```python
from build123d import *

# Parameters (mm, degrees)
BOSS_EXTRUDE1_DEPTH                             = 182.5
CUT_EXTRUDE1_DEPTH                              = 251
CUT_EXTRUDE2_DEPTH                              = 10
SKETCH4_W                                       = 2
SKETCH4_H                                       = 246
BOSS_EXTRUDE2_DEPTH                             = 43
SKETCH5_W                                       = 3
SKETCH5_H                                       = 3
CUT_EXTRUDE3_DEPTH                              = 46
FILLET1_R                                       = 0.5
FILLET2_R                                       = 2.5
CUT_EXTRUDE6_DEPTH                              = 366
SKETCH9_R                                       = 2.25
CUT_EXTRUDE7_DEPTH                              = 366
SKETCH10_R                                      = 2.25
CUT_EXTRUDE8_DEPTH                              = 10
SKETCH11_R                                      = 2.25
CUT_EXTRUDE9_DEPTH                              = 10
SKETCH12_R                                      = 1.5
CUT_EXTRUDE10_DEPTH                             = 10
CSK_FOR_M3_FLAT_HEAD_MACHINE_SCREW1_D           = 3.4
CSK_FOR_M3_FLAT_HEAD_MACHINE_SCREW1_CSINK_D     = 6.3
CSK_FOR_M3_FLAT_HEAD_MACHINE_SCREW1_CSINK_ANGLE = 90


with BuildPart() as part:
    # Sketch1 → Boss-Extrude1 (new body, symmetric)
    with BuildSketch(Plane(origin=(0, 0, 0), x_dir=(0, 0, -1), z_dir=(1, 0, 0))):
        with BuildLine():
            Line((123, -45), (125, -45))
            Line((125, -45), (125, -2.5))
            ThreePointArc((125, -2.5), (124.267766953, -0.732233047), (122.5, 0))
            Line((122.5, 0), (-122.5, 0))
            ThreePointArc((-122.5, 0), (-124.267766953, -0.732233047), (-125, -2.5))
            Line((-125, -2.5), (-125, -45))
            Line((-125, -45), (-123, -45))
            Line((-123, -45), (-123, -2.5))
            ThreePointArc((-123, -2.5), (-122.853553391, -2.146446609), (-122.5, -2))
            Line((-122.5, -2), (122.5, -2))
            ThreePointArc((122.5, -2), (122.853553391, -2.146446609), (123, -2.5))
            Line((123, -2.5), (123, -45))
        make_face()
    extrude(amount=BOSS_EXTRUDE1_DEPTH, both=True)

    # Sketch2 → Cut-Extrude1 (cut, through all)
    with BuildSketch(Plane.XY.offset(125)):
        with BuildLine():
            Line((-164.5, -45), (164.5, -45))
            Line((164.5, -45), (164.5, -28))
            ThreePointArc((164.5, -28), (161.571067812, -20.928932188), (154.5, -18))
            Line((154.5, -18), (-154.5, -18))
            ThreePointArc((-154.5, -18), (-161.571067812, -20.928932188), (-164.5, -28))
            Line((-164.5, -28), (-164.5, -45))
        make_face()
    extrude(amount=-CUT_EXTRUDE1_DEPTH, mode=Mode.SUBTRACT)

    # Sketch3 → Cut-Extrude2 (cut)
    with BuildSketch(Plane(origin=(0, 0, 0), x_dir=(1, 0, 0), z_dir=(0, 1, 0))):
        with BuildLine():
            Line((-117.5, 105), (117.5, 105))
            ThreePointArc((117.5, 105), (131.642135624, 99.142135624), (137.5, 85))
            Line((137.5, 85), (137.5, -45))
            ThreePointArc((137.5, -45), (131.642135624, -59.142135624), (117.5, -65))
            Line((117.5, -65), (-117.5, -65))
            ThreePointArc((-117.5, -65), (-131.642135624, -59.142135624), (-137.5, -45))
            Line((-137.5, -45), (-137.5, 85))
            ThreePointArc((-137.5, 85), (-131.642135624, 99.142135624), (-117.5, 105))
        make_face()
    extrude(amount=-CUT_EXTRUDE2_DEPTH, mode=Mode.SUBTRACT)

    # Sketch4 → Boss-Extrude2 (add)
    with BuildSketch(Plane.XZ.offset(2)):
        with Locations((-181.5, 0)):
            Rectangle(SKETCH4_W, SKETCH4_H)
        with Locations((181.5, 0)):
            Rectangle(SKETCH4_W, SKETCH4_H)
    extrude(amount=BOSS_EXTRUDE2_DEPTH)

    # Sketch5 → Cut-Extrude3 (cut, through all)
    with BuildSketch(Plane.XZ.offset(45)):
        with Locations((-181, 123.5)):
            Rectangle(SKETCH5_W, SKETCH5_H)
        with Locations((-181, -123.5)):
            Rectangle(SKETCH5_W, SKETCH5_H)
        with Locations((181, -123.5)):
            Rectangle(SKETCH5_W, SKETCH5_H)
        with Locations((181, 123.5)):
            Rectangle(SKETCH5_W, SKETCH5_H)
    extrude(amount=-CUT_EXTRUDE3_DEPTH, mode=Mode.SUBTRACT)

    # Fillet1
    fillet1_edges = [part.edges().sort_by_distance(p)[0] for p in [
        (-180.5, -2, 0),
        (180.5, -2, 0),
    ]]
    fillet(fillet1_edges, radius=FILLET1_R)

    # Fillet2
    fillet2_edges = [part.edges().sort_by_distance(p)[0] for p in [
        (-182.5, 0, 0),
        (182.5, 0, 0),
    ]]
    fillet(fillet2_edges, radius=FILLET2_R)

    # Sketch8 → Cut-Extrude6 (cut, through all)
    with BuildSketch(Plane.ZY.offset(182.5)):
        with BuildLine():
            Line((-107, -45), (107, -45))
            Line((107, -45), (107, -11))
            ThreePointArc((107, -11), (105.535533906, -7.464466094), (102, -6))
            Line((102, -6), (-102, -6))
            ThreePointArc((-102, -6), (-105.535533906, -7.464466094), (-107, -11))
            Line((-107, -11), (-107, -45))
        make_face()
    extrude(amount=-CUT_EXTRUDE6_DEPTH, mode=Mode.SUBTRACT)

    # Sketch9 → Cut-Extrude7 (cut, through all)
    with BuildSketch(Plane.ZY.offset(182.5)):
        with Locations((-118, -9)):
            Circle(SKETCH9_R)
        with Locations((-118, -33)):
            Circle(SKETCH9_R)
        with Locations((118, -9)):
            Circle(SKETCH9_R)
        with Locations((118, -33)):
            Circle(SKETCH9_R)
    extrude(amount=-CUT_EXTRUDE7_DEPTH, mode=Mode.SUBTRACT)

    # Sketch10 → Cut-Extrude8 (cut)
    with BuildSketch(Plane.XY.offset(125)):
        with Locations((-151.5, -9)):
            Circle(SKETCH10_R)
        with Locations((175.5, -21)):
            Circle(SKETCH10_R)
        with Locations((151.5, -9)):
            Circle(SKETCH10_R)
        with Locations((-175.5, -21)):
            Circle(SKETCH10_R)
    extrude(amount=-CUT_EXTRUDE8_DEPTH, mode=Mode.SUBTRACT)

    # Sketch11 → Cut-Extrude9 (cut)
    with BuildSketch(Plane(origin=(0, 0, -125), x_dir=(-1, 0, 0), z_dir=(0, 0, -1))):
        with Locations(Location((-175.5, -21, 0), (0, 0, 180))):  # turned: the seam where the file's is
            Circle(SKETCH11_R)
        with Locations(Location((-151.5, -9, 0), (0, 0, 180))):  # turned: the seam where the file's is
            Circle(SKETCH11_R)
        with Locations(Location((151.5, -9, 0), (0, 0, 180))):  # turned: the seam where the file's is
            Circle(SKETCH11_R)
        with Locations(Location((175.5, -21, 0), (0, 0, 180))):  # turned: the seam where the file's is
            Circle(SKETCH11_R)
    extrude(amount=-CUT_EXTRUDE9_DEPTH, mode=Mode.SUBTRACT)

    # Sketch12 → Cut-Extrude10 (cut)
    with BuildSketch(Plane(origin=(0, 0, 0), x_dir=(1, 0, 0), z_dir=(0, 1, 0))):
        with Locations(Location((-45, -79, 0), (0, 0, 270))):  # turned: the seam where the file's is
            Circle(SKETCH12_R)
        with Locations(Location((17.5, -79, 0), (0, 0, 270))):  # turned: the seam where the file's is
            Circle(SKETCH12_R)
        with Locations(Location((-107.5, -79, 0), (0, 0, 270))):  # turned: the seam where the file's is
            Circle(SKETCH12_R)
        with Locations(Location((-157.5, -108, 0), (0, 0, 270))):  # turned: the seam where the file's is
            Circle(SKETCH12_R)
        with Locations(Location((-157.5, -118, 0), (0, 0, 270))):  # turned: the seam where the file's is
            Circle(SKETCH12_R)
        with Locations(Location((27.5, -108, 0), (0, 0, 270))):  # turned: the seam where the file's is
            Circle(SKETCH12_R)
        with Locations(Location((27.5, -118, 0), (0, 0, 270))):  # turned: the seam where the file's is
            Circle(SKETCH12_R)
    extrude(amount=-CUT_EXTRUDE10_DEPTH, mode=Mode.SUBTRACT)

    # CSK for M3 Flat Head Machine Screw1 (through all)
    with Locations(Plane(origin=(0, 0, 0), x_dir=(-1, 0, 0), z_dir=(0, 1, 0))):
        with Locations((107.5, 79), (45, 79), (-17.5, 79), (157.5, 108), (157.5, 118), (-27.5, 108), (-27.5, 118)):
            CounterSinkHole(CSK_FOR_M3_FLAT_HEAD_MACHINE_SCREW1_D / 2, CSK_FOR_M3_FLAT_HEAD_MACHINE_SCREW1_CSINK_D / 2, counter_sink_angle=CSK_FOR_M3_FLAT_HEAD_MACHINE_SCREW1_CSINK_ANGLE)


solid = part.part
```
The listing builds one solid part. Answer for the finished solid, in the listing's coordinates (mm). A direction names the side the tool comes from. Give positions to 0.01 mm unless a question says otherwise; leave off trailing zeros. Order: outer loops, then holes, each group sorted by start corner. A loop starts at its lowest first (then second) coordinate and runs counter-clockwise, first axis right, second up. Notation, with made-up numbers: (-23.5, -10) -> (14.5, -10) arc R25 cw to (14.5, 24) -> close; hole circle Ø2 at (70.5, 77.25). An arc over 180 degrees is marked (long way). One line per item, written item: value.
1) Find section C-C, the plane x = -143. Determine the outline of the cut face in (y, z), plus the area to 3 significant figures.
Reported:
outline: (-18, -125) -> (-2.5, -125) arc R2.5 ccw to (0, -122.5) -> (0, 122.5) arc R2.5 ccw to (-2.5, 125) -> (-18, 125) -> (-18, 123) -> (-2.5, 123) arc R0.5 cw to (-2, 122.5) -> (-2, -122.5) arc R0.5 cw to (-2.5, -123) -> (-18, -123) -> close
area: 561 mm^2
2) Find section A-A, the plane z = 22.5. Determine the outline of the cut face in (x, y), plus the area to 3 significant figures.
Reported:
outline: (-182.5, -6) -> (-180.5, -6) -> (-180.5, -2.5) arc R0.5 cw to (-180, -2) -> (-137.5, -2) -> (-137.5, 0) -> (-180, 0) arc R2.5 ccw to (-182.5, -2.5) -> close; (137.5, -2) -> (180, -2) arc R0.5 cw to (180.5, -2.5) -> (180.5, -6) -> (182.5, -6) -> (182.5, -2.5) arc R2.5 ccw to (180, 0) -> (137.5, 0) -> close
area: 193 mm^2
3) Determine the mould class of faces 1 (the flat face through (-12, -7, -125)), 2 (the cylindrical face through (131.486, -0.986, -99.297)), 3 (the cylindrical face through (-161.49, -20.85, -123.99)) for opening direction Z: pulls with the +Z half, pulls with the -Z half, needs draft (parallel to the pull), parting line crosses it, or undercut.
Reported:
face 1: pulls with the -Z half
face 2: undercut
face 3: needs draft
4) Flat-ended cylindrical pins translate along their axes: P1, Ø1, axis at x = 181.5, z = -26.5, coming from the -Y side; P2, Ø0.6, axis at x = -181.5, y = -20.5, coming from the -Z side; P3, Ø1.6, axis at x = 181, y = -23, coming from the +Z side. Find the tip coordinate at first contact, or state that the pin passes through.
Reported:
P1: stops at y = -6
P2: stops at z = -122
P3: stops at z = 122
5) Find the intervals of material crossed by line 1 (Z direction, x = 166, y = -33.5); line 2 (Y direction, x = -157, z = 25.5); line 3 (Y direction, x = 181, z = 118), in increasing order.
Reported:
line 1: z = -125 to -123, 123 to 125
line 2: y = -2 to 0
line 3: y = -45 to -35.25, -30.75 to -11.25, -6.75 to -0.21
6) A tool of negligible diameter and unlimited length cuts with its end or side. For faces 4 (the cylindrical face through (-161.49, -20.85, 124.01)), 5 (the flat face through (1, -5, -123)), 6 (the flat face through (3, 0, 80)), 7 (the flat face through (3, -2, 83)), 8 (the cylindrical face through (-131.797, -0.986, -98.986)), from which of +Z, -Z, +X, -X, +Y, -Y can it reach the whole face along a straight path? Write none if from no direction.
Reported:
face 4: +Z, -Z, -Y
face 5: +X, -X, -Y
face 6: +Z, -Z, +X, -X, +Y
face 7: -Y
face 8: +Y, -Y
7) Find section B-B, the plane x = 85.5. Determine the outline of the cut face in (y, z).
Reported:
outline: (-18, -125) -> (-2.5, -125) arc R2.5 ccw to (0, -122.5) -> (0, -105) -> (-2, -105) -> (-2, -122.5) arc R0.5 cw to (-2.5, -123) -> (-18, -123) -> close; (-18, 123) -> (-2.5, 123) arc R0.5 cw to (-2, 122.5) -> (-2, 65) -> (0, 65) -> (0, 122.5) arc R2.5 ccw to (-2.5, 125) -> (-18, 125) -> close
